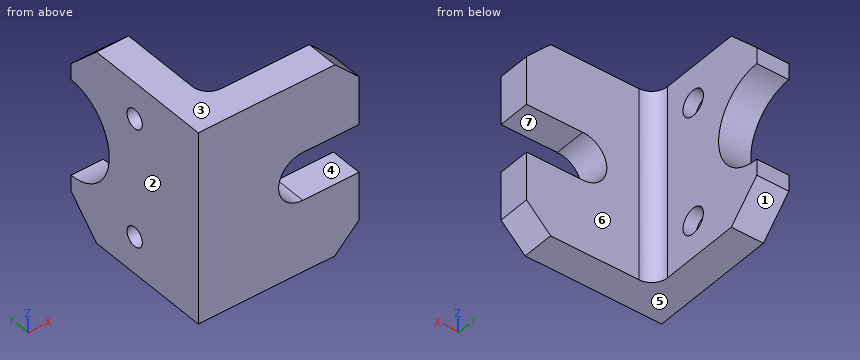
```python
from build123d import *

# Parameters (mm, degrees)
BOSS_EXTRUDE1_DEPTH     = 60
CHAMFER1_SIZE           = 15
CHAMFER2_SIZE           = 20
FILLET2_R               = 10
CUT_EXTRUDE1_REACH      = 143.421
SKETCH2_R               = 6
SKETCH2_3_R             = 8
SKETCH2_3_R_2           = 6
CUT_EXTRUDE2_DEPTH      = 8
CUT_EXTRUDE3_DEPTH      = 142.421356237
CUT_EXTRUDE3_DEPTH_BACK = 20


with BuildPart() as part:
    # Sketch1 → Boss-Extrude1 (new, symmetric)
    with BuildSketch(Plane.XY):
        Polygon((0, 0), (100, 0), (100, 20), (20, 20), (20, 100), (0, 100), align=None)
    extrude(amount=BOSS_EXTRUDE1_DEPTH, both=True)

    # Chamfer1
    chamfer1_edges = [part.edges().sort_by_distance(p)[0] for p in [
        (100, 10, 60),
        (100, 10, -60),
    ]]
    chamfer(chamfer1_edges, length=CHAMFER1_SIZE)

    # Chamfer2
    chamfer2_edges = [part.edges().sort_by_distance(p)[0] for p in [
        (10, 100, 60),
        (10, 100, -60),
    ]]
    chamfer(chamfer2_edges, length=CHAMFER2_SIZE)

    # Fillet2
    fillet2_edges = [part.edges().sort_by_distance(p)[0] for p in [
        (20, 20, 0),
    ]]
    fillet(fillet2_edges, radius=FILLET2_R)

    # Sketch2 → Cut-Extrude1 (cut, up to next)
    with BuildSketch(Plane(origin=(20, 0, 0), x_dir=(0, 0, -1), z_dir=(1, 0, 0)), mode=Mode.PRIVATE) as cut_extrude1_sk1:
        with BuildLine():
            Line((30, 100), (-30, 100))
            ThreePointArc((-30, 100), (0, 70), (30, 100))
        make_face()
    cut_extrude1_tool1 = extrude(cut_extrude1_sk1.sketch, amount=-CUT_EXTRUDE1_REACH, mode=Mode.PRIVATE) & part.part
    # Sketch2 → Cut-Extrude1 (cut, up to next)
    with BuildSketch(Plane(origin=(20, 0, 0), x_dir=(0, 0, -1), z_dir=(1, 0, 0)), mode=Mode.PRIVATE) as cut_extrude1_sk2:
        with Locations(Location((37, 50, 0), (0, 0, 90))):
            Circle(SKETCH2_R)
    cut_extrude1_tool2 = extrude(cut_extrude1_sk2.sketch, amount=-CUT_EXTRUDE1_REACH, mode=Mode.PRIVATE) & part.part
    # Sketch2 → Cut-Extrude1 (cut, up to next)
    with BuildSketch(Plane(origin=(20, 0, 0), x_dir=(0, 0, -1), z_dir=(1, 0, 0)), mode=Mode.PRIVATE) as cut_extrude1_sk3:
        with Locations(Location((-37, 50, 0), (0, 0, 90))):
            Circle(SKETCH2_R)
    cut_extrude1_tool3 = extrude(cut_extrude1_sk3.sketch, amount=-CUT_EXTRUDE1_REACH, mode=Mode.PRIVATE) & part.part
    add(cut_extrude1_tool1.solids().sort_by_distance((20, 87.267605, 0))[0], mode=Mode.SUBTRACT)
    add(cut_extrude1_tool2.solids().sort_by_distance((20, 50, -37))[0], mode=Mode.SUBTRACT)
    add(cut_extrude1_tool3.solids().sort_by_distance((20, 50, 37))[0], mode=Mode.SUBTRACT)

    # Sketch2_3 → Cut-Extrude2 (cut)
    # profile 1 of 2: a face of its own
    with BuildSketch(Plane(origin=(20, 0, 0), x_dir=(0, 0, -1), z_dir=(1, 0, 0))):
        with Locations(Location((37, 50, 0), (0, 0, 90))):
            Circle(SKETCH2_3_R)
        with Locations(Location((37, 50, 0), (0, 0, 90))):
            Circle(SKETCH2_3_R_2, mode=Mode.SUBTRACT)
    # profile 2 of 2: a face of its own
    with BuildSketch(Plane(origin=(20, 0, 0), x_dir=(0, 0, -1), z_dir=(1, 0, 0))):
        with Locations(Location((-37, 50, 0), (0, 0, 90))):
            Circle(SKETCH2_3_R)
        with Locations(Location((-37, 50, 0), (0, 0, 90))):
            Circle(SKETCH2_3_R_2, mode=Mode.SUBTRACT)
    extrude(amount=-CUT_EXTRUDE2_DEPTH, mode=Mode.SUBTRACT)

    # Sketch3 → Cut-Extrude3 (cut, two sides: drawn at the far end of the back side and taken through both)
    with BuildSketch(Plane(origin=(0, 20, 0), x_dir=(1, 0, 0), z_dir=(0, 1, 0)).offset(-CUT_EXTRUDE3_DEPTH_BACK)):
        with BuildLine():
            Line((360, 15), (100, 15))
            Line((100, 15), (65, 15))
            ThreePointArc((65, 15), (50, 0), (65, -15))
            Line((65, -15), (100, -15))
            Line((100, -15), (360, -15))
            Line((360, -15), (880, -15))
            Line((880, -15), (880, 15))
            Line((880, 15), (360, 15))
        make_face()
    extrude(amount=CUT_EXTRUDE3_DEPTH + CUT_EXTRUDE3_DEPTH_BACK, mode=Mode.SUBTRACT)


solid = part.part
```
Geometry check sheet. Reference: the model listing, model coordinates, mm. Face numbers are marked on the shaded views. A direction names the side the tool comes from. Round coordinates to 2 decimals unless told otherwise and drop trailing zeros. Order: outer loops, then holes, each group sorted by start corner. A loop starts at its lowest first (then second) coordinate and runs counter-clockwise, first axis right, second up. Notation, with made-up numbers: (23, 81) - (59, 81) arc R10 cw to (59, 100) - close; hole circle Ø2 at (68.5, -10). An arc over 180 degrees is marked (long way). Use a Markdown table: item, result. Add a question column.
(1) Tool access check on the marked faces 5, 6 and 7. Record the directions out of +Z, -Z, +X, -X, +Y, -Y that give a thin tool (end or side, any length) a straight path to the whole face; none if there is none.
(2) Material ranges on line 1 along Z through (x, y) = (5, 50); line 2 along Z through (x, y) = (7.5, 78); line 3 along X through (y, z) = (59, -42), recorded low to high. Write a range as [from, to].
(3) Sectioned sample at A-A, the plane z = 37. Enter the section's corners in (x, y), and give its area (3 significant figures).
(4) Release check for a two-part mould opening along Z. For the marked faces 1, 2, 3 and 4 record: pulls with the +Z half, pulls with the -Z half, needs draft (parallel to the pull), parting line crosses it, or undercut.
(5) Sectioned sample at D-D, the plane z = 0. Enter the section's corners in (x, y), and give its area (3 significant figures).
(6) Sectioned sample at C-C, the plane x = 8. Enter the section's corners in (y, z).
(7) Depth check by flat-ended pin: pin 1 (8 mm diameter, centred on x = 61, z = -30, fed in from +Y); pin 2 (17.5 mm diameter, centred on y = 49.5, z = 36.5, fed in from +X); pin 3 (13 mm diameter, centred on y = 51, z = -38, fed in from +X). Enter the tip coordinate at first touch or a pass-through.
(8) Sectioned sample at B-B, the plane y = 50. Enter the section's corners in (x, z).
Answers below:
| question | item | result |
|---|---|---|
| 1 | face 5 | -Z, +X, -X, +Y, -Y |
| 1 | face 6 | +Z, -Z, +X, +Y |
| 1 | face 7 | +X, +Y, -Y |
| 2 | line 1 | [-60, -43], [-31, 31], [43, 60] |
| 2 | line 2 | [-60, -20.4], [20.4, 60] |
| 2 | line 3 | [0, 20] |
| 3 | outline | (0, 0) - (100, 0) - (100, 20) - (30, 20) arc R10 cw to (20, 30) - (20, 42) - (12, 42) - (12, 44) - (0, 44) - close; (0, 56) - (12, 56) - (12, 58) - (20, 58) - (20, 100) - (0, 100) - close |
| 3 | area | 3,350 mm² |
| 4 | face 1 | pulls with the -Z half |
| 4 | face 2 | needs draft |
| 4 | face 3 | pulls with the +Z half |
| 4 | face 4 | undercut |
| 5 | outline | (0, 0) - (50, 0) - (50, 20) - (30, 20) arc R10 cw to (20, 30) - (20, 70) - (0, 70) - close |
| 5 | area | 2,020 mm² |
| 6 | outline | (0, -60) - (80, -60) - (100, -40) - (100, -30) arc R30 cw to (100, 30) - (100, 40) - (80, 60) - (0, 60) - close; hole circle Ø12 at (50, -37); hole circle Ø12 at (50, 37) |
| 7 | pin 1 | y = 20 |
| 7 | pin 2 | x = 20 |
| 7 | pin 3 | x = 12 |
| 8 | outline | (0, -60) - (20, -60) - (20, -45) - (12, -45) - (12, -43) - (0, -43) - close; (0, -31) - (12, -31) - (12, -29) - (20, -29) - (20, 29) - (12, 29) - (12, 31) - (0, 31) - close; (0, 43) - (12, 43) - (12, 45) - (20, 45) - (20, 60) - (0, 60) - close |
